Study the drawing (mm; zero at the part's minimum x, y, z) and answer. A direction names the side the tool comes from. Coordinates: 2 decimals unless noted, no trailing zeros. Write each loop counter-clockwise with the first axis right and the second up, starting at its lowest first coordinate (ties: lowest second). Pieces come first, ordered by that corner, then holes. Notation, with made-up numbers: M -3.5,-30 L 52.5,-30 A18 ccw 52.5,-11 Z; hole C 23,-3.5 d7. An arc over 180 degrees is marked long. Answer as a JSON object with one key per item and string values. Group by question number.
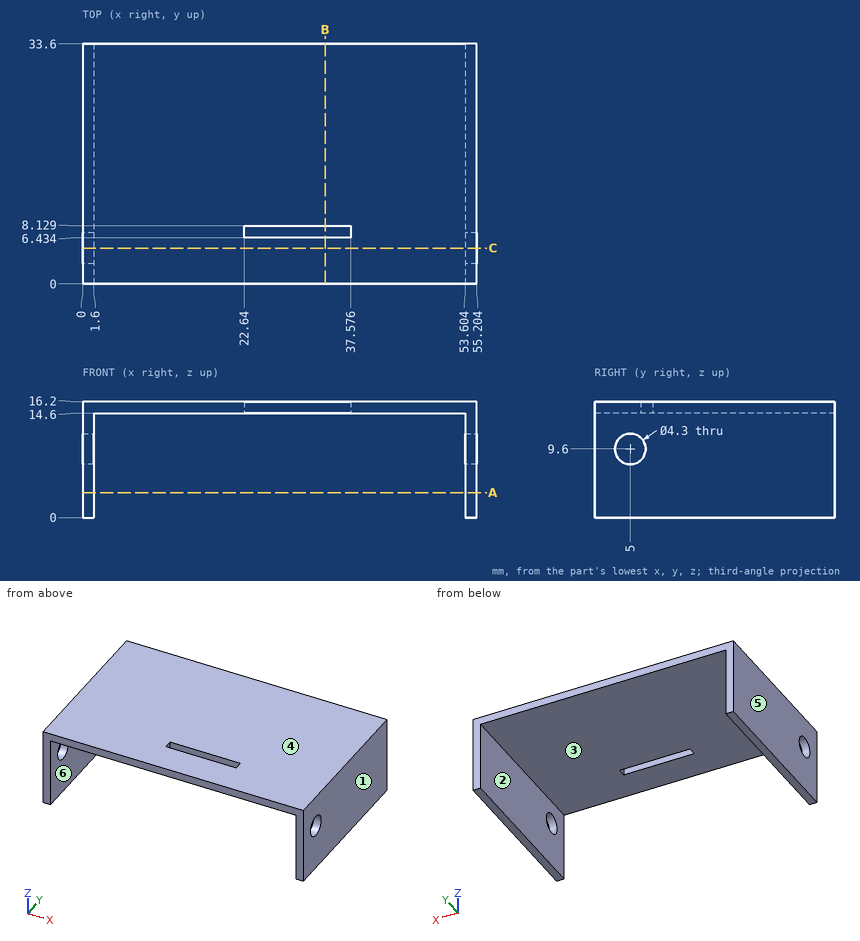
Item 1: Flat-ended cylindrical pins translate along their axes: pin 1 Ø1 at (x, y) = (9, 17) entering from -Z; pin 2 Ø1.3 at (x, z) = (33.5, 15.5) entering from -Y. Find the tip coordinate at first contact, or state that the pin passes through.
Item 2: A cutting plane is placed at B-B, the plane x = 34. Write down the section's boundary in (y, z).
Item 3: Consider L1, parallel to X at y = 25, z = 12 (1 decimal); L2, parallel to Y at x = 0.85, z = 9.6; L3, parallel to Z at x = 54.65, y = 5. Determine where each line is inside the solid, lowest interval first. Write a range as from..to.
Item 4: For a pull along X with two mould halves and no side action, classify the marked faces 3, 4, 5 and 6 as +X half, -X half, draft (parallel to the pull), parting line (faces both ways), or undercut.
Item 5: A cutting plane is placed at A-A, the plane z = 3.5. Write down the section's boundary in (x, y) (1 decimal).
Item 6: A tool of negligible diameter and unlimited length cuts with its end or side. For the marked faces 1 and 2, from which of +Z, -Z, +X, -X, +Y, -Y can it reach the whole face along a straight path? Write none if from no direction.
Item 7: A cutting plane is placed at C-C, the plane y = 5. State how many separate pieces and enclosed holes the cut face has, and give its area (3 significant figures).
Answer:
{
 "1": {"pin 1": "z = 14.6", "pin 2": "y = 0"},
 "2": {"outline": "M 0,14.6 L 6.43,14.6 L 6.43,16.2 L 0,16.2 Z; M 8.13,14.6 L 33.6,14.6 L 33.6,16.2 L 8.13,16.2 Z"},
 "3": {"L1": "0..1.6, 53.6..55.2", "L2": "0..2.85, 7.15..33.6", "L3": "0..7.45, 11.75..16.2"},
 "4": {"face 3": "undercut", "face 4": "draft", "face 5": "-X half", "face 6": "undercut"},
 "5": {"outline": "M 0,0 L 1.6,0 L 1.6,33.6 L 0,33.6 Z; M 53.6,0 L 55.2,0 L 55.2,33.6 L 53.6,33.6 Z"},
 "6": {"face 1": "+Z, -Z, +X, +Y, -Y", "face 2": "-Z, +Y, -Y"},
 "7": {"separate pieces": "3", "enclosed holes": "0", "area": "121 mm2"}
}
